from build123d import *

# Parameters (mm, degrees)
F0_R      = 25
F0_R_2    = 22.5
F1_DEPTH  = 5
F3_R      = 1.25
F4_DEPTH  = 3.8
F6_R      = 1.25
F7_DEPTH  = 3.4
F8_R      = 1.25
F9_DEPTH  = 0.25
F10_R     = 1.25
F11_DEPTH = 0.25
F13_R     = 1.25
F13_R_2   = 1.1
F14_DEPTH = 25
F16_R     = 1.25
F17_DEPTH = 4.4


# Not quite as in the source:
# - a pattern or mirror of a feature is missing from the dataset's text; its kind, count and spacing are read off the source's solid


with BuildPart() as f1:
    # F0 (on Front) → F1 (new body)
    with BuildSketch(Plane.XZ):
        Circle(F0_R)
        Circle(F0_R_2, mode=Mode.SUBTRACT)
    extrude(amount=F1_DEPTH)

    # F3 (on offset) → F4 (join)
    with BuildSketch(Plane.XY.offset(24.83)):
        with Locations((0, -2.5)):
            Circle(F3_R)
    extrude(amount=F4_DEPTH)

    # F6 (on offset) → F7 (join)
    with BuildSketch(Plane.XY.offset(-24.39)):
        with Locations((0, -2.5)):
            Circle(F6_R)
    extrude(amount=-F7_DEPTH)

    # F8 (on face) → F9 (join)
    with BuildSketch(Plane(origin=(0, 0, -27.79), x_dir=(1, 0, 0), z_dir=(0, 0, -1))):
        with Locations((0, 2.5)):
            Circle(F8_R)
    extrude(amount=F9_DEPTH)

    # F10 (on face) → F11 (join)
    with BuildSketch(Plane.XY.offset(28.63)):
        with Locations((0, -2.5)):
            Circle(F10_R)
    extrude(amount=F11_DEPTH)

    # F13 (on offset) → F14 (cut)
    with BuildSketch(Plane.XY.offset(24.83)):
        with Locations((0, -2.5)):
            Circle(F13_R)
        with Locations((0, -2.5)):
            Circle(F13_R_2, mode=Mode.SUBTRACT)
    extrude(amount=F14_DEPTH, mode=Mode.SUBTRACT)

    # F16 (on offset) → F17 (join)
    with BuildSketch(Plane.YZ.offset(23.5)):
        with Locations((-2.5, 0)):
            Circle(F16_R)
    f17 = extrude(amount=-F17_DEPTH)

    # F17_copies: F17 across plane
    add(f17.mirror(Plane(origin=(0, 0, 0), x_dir=(0, 0, -1), z_dir=(-1, 0, 0))))


solid = f1.part
The listing builds one solid part. Answer for the finished solid, in the listing's coordinates (mm). A direction names the side the tool comes from. Give positions to 0.01 mm unless a question says otherwise; leave off trailing zeros. Write each loop counter-clockwise with the first axis right and the second up, starting at its lowest first coordinate (ties: lowest second). Pieces come first, ordered by that corner, then holes. Notation, with made-up numbers: (0.25, 52) -> (27.25, 52) arc R26 cw to (27.25, 75) -> close; hole circle Ø11 at (73, 38). An arc over 180 degrees is marked (long way). One line per question, with ' | ' between items. Start each with the question number.
1. For a pull along X with two mould halves and no side action, classify faces 1 (the cylindrical face through (23.846, -2.465, 7.509)), 2 (the flat face through (-22.34, -5, 3.82)), 3 (the flat face through (19.1, -3, 0)) as pulls with the +X half, pulls with the -X half, needs draft (parallel to the pull), parting line crosses it, or undercut.
2. Section D-D (x = 21.5) is taken. Determine the outline of the cut face in (y, z).
3. Given pin 1 Ø2 at (x, y) = (-10, -3) entering from -Z; pin 2 Ø1.5 at (x, y) = (6, -3) entering from +Z; pin 3 Ø1 at (y, z) = (-2.5, -9) entering from -X, each flat-ended and moving along its own axis, determine where each tip first touches the part or whether it passes through.
4. For faces 4 (the cylindrical face through (20.82, -1.31, 0.38)), 5 (the flat face through (-19.1, -3, 0)), 6 (the cylindrical face through (-0.16, -1.26, -26.48)), 7 (the cylindrical face through (0.59, -1.57, 26.83)), determine the directions among +Z, -Z, +X, -X, +Y, -Y from which every point of the face is accessible in a straight line to the end or side of a thin tool.
5. Section B-B (z = 0) is taken. Determine the outline of the cut face in (x, y), plus the area to 3 significant figures.
6. Section A-A (x = -5) is taken. Determine the outline of the cut face in (y, z), plus the area to 3 significant figures.
7. Find the intervals of material crossed by probe 1 along Y at (x, z) = (0, 24.9); probe 2 along Z at (x, y) = (0, -3.4); probe 3 along Z at (x, y) = (8, -0.55), in increasing order.
Response values:
1) face 1: parting line crosses it | face 2: needs draft | face 3: undercut
2) outline: (-5, -12.76) -> (0, -12.76) -> (0, -6.63) -> (-5, -6.63) -> close; (-5, 6.63) -> (0, 6.63) -> (0, 12.76) -> (-5, 12.76) -> close; circle Ø2.5 at (-2.5, 0)
3) pin 1: z = -23.32 | pin 2: z = 24.44 | pin 3: x = -23.51
4) face 4: none | face 5: +Y, -Y | face 6: -Z | face 7: +Z
5) outline: (-25, -5) -> (-22.5, -5) -> (-22.5, -3.75) -> (-19.1, -3.75) -> (-19.1, -1.25) -> (-22.5, -1.25) -> (-22.5, 0) -> (-25, 0) -> close; (19.1, -3.75) -> (22.5, -3.75) -> (22.5, -5) -> (25, -5) -> (25, 0) -> (22.5, 0) -> (22.5, -1.25) -> (19.1, -1.25) -> close | area: 42.0 mm2
6) outline: (-5, -24.49) -> (0, -24.49) -> (0, -21.94) -> (-5, -21.94) -> close; (-5, 21.94) -> (0, 21.94) -> (0, 24.49) -> (-5, 24.49) -> close | area: 25.6 mm2
7) probe 1: -5 to -3.75, -3.6 to -1.4, -1.25 to 0 | probe 2: -28.04 to -22.5, 22.5 to 28.88 | probe 3: -23.69 to -21.03, 21.03 to 23.69
